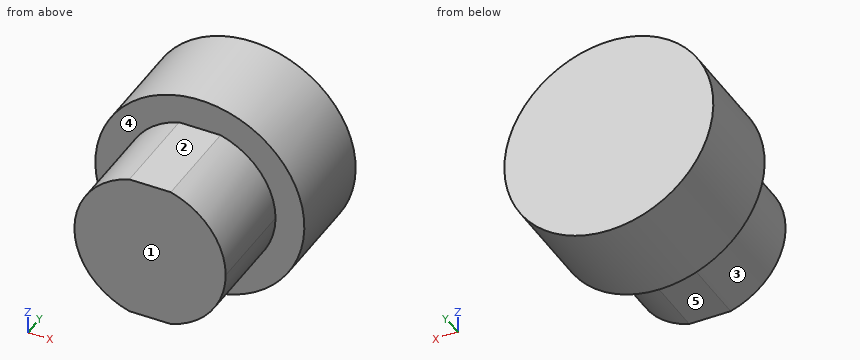
from build123d import *

# Parameters (mm, degrees)
BOSS_EXTRUDE1_DEPTH = 13.3
SKETCH2_R           = 14.5
BOSS_EXTRUDE2_DEPTH = 13.7


with BuildPart() as part:
    # Sketch1 → Boss-Extrude1 (new body)
    with BuildSketch(Plane(origin=(0, 0, 0), x_dir=(1, 0, 0), z_dir=(0, 1, 0))):
        with BuildLine():
            Line((2.870540019, 10.1), (-2.870540019, 10.1))
            ThreePointArc((-2.870540019, 10.1), (-10.5, 0), (-2.870540019, -10.1))
            Line((-2.870540019, -10.1), (2.870540019, -10.1))
            Line((2.870540019, -10.1), (2.870540019, 10.1))
        make_face()
        with BuildLine():
            ThreePointArc((10.5, 0), (8.378265638, 6.328875485), (2.870540019, 10.1))
            Line((2.870540019, 10.1), (2.870540019, -10.1))
            ThreePointArc((2.870540019, -10.1), (8.378265638, -6.328875485), (10.5, 0))
        make_face()
    extrude(amount=BOSS_EXTRUDE1_DEPTH)

    # Sketch2 → Boss-Extrude2 (add)
    with BuildSketch(Plane(origin=(0, 13.3, 0), x_dir=(1, 0, 0), z_dir=(0, 1, 0))):
        with Locations(Location((0, 0, 0), (0, 0, 90))):
            Circle(SKETCH2_R)
    extrude(amount=BOSS_EXTRUDE2_DEPTH)


solid = part.part
Can you work these out from the model? Positions are in its coordinate system, mm. Face numbers are marked on the shaded views. A direction names the side the tool comes from. Round coordinates to 2 decimals unless told otherwise and drop trailing zeros. Order: outer loops, then holes, each group sorted by start corner. A loop starts at its lowest first (then second) coordinate and runs counter-clockwise, first axis right, second up. Notation, with made-up numbers: M 42,34 L 65,34 A11 cw 65,53 Z; hole C 11.25,15 d9. An arc over 180 degrees is marked long. Use a Markdown table: item, result.
1) Imagine slicing it at D-D (y = 19). List the corners of the cut face in (x, z) for me, then the cut area to 3 significant figures.
Geometry says:
| item | result |
|---|---|
| outline | C 0,0 d29 |
| area | 661 mm² |
2) Imagine slicing it at C-C (y = 3.75). List the corners of the cut face in (x, z) for me, then the cut area to 3 significant figures.
Geometry says:
| item | result |
|---|---|
| outline | M -2.87,-10.1 L 2.87,-10.1 A10.5 ccw 2.87,10.1 L -2.87,10.1 A10.5 ccw Z |
| area | 343 mm² |
3) I'm going to push flat-ended pins straight in: P1, Ø10, axis at y = 7, z = 8, coming from the +X side; P2, Ø6.5, axis at x = 1, y = 4, coming from the -Z side; P3, Ø2, axis at y = 4, z = -4.5, coming from the +X side. Where does each tip first touch, or does it pass through?
Geometry says:
| item | result |
|---|---|
| P1 | stops at x = 10.06 |
| P2 | stops at z = -10.1 |
| P3 | stops at x = 9.9 |
4) If I drill on line 1 along Y through (x, z) = (7.25, 10.75); line 2 along Z through (x, y) = (1.75, 5.5); line 3 along X through (y, z) = (10.75, 0), over which ranges is the centre line in solid material (lowest first)?
Geometry says:
| item | result |
|---|---|
| line 1 | y = 13.3 to 27 |
| line 2 | z = -10.1 to 10.1 |
| line 3 | x = -10.5 to 10.5 |
5) Imagine slicing it at B-B (z = -6.5). List the corners of the cut face in (x, y) for me, then the cut area to 3 significant figures.
Geometry says:
| item | result |
|---|---|
| outline | M -12.96,13.3 L -8.25,13.3 L -8.25,0 L 8.25,0 L 8.25,13.3 L 12.96,13.3 L 12.96,27 L -12.96,27 Z |
| area | 574 mm² |
6) Imagine slicing it at A-A (x = 0). List the corners of the cut face in (y, z) for me, then the cut area to 3 significant figures.
Geometry says:
| item | result |
|---|---|
| outline | M 0,-10.1 L 13.3,-10.1 L 13.3,-14.5 L 27,-14.5 L 27,14.5 L 13.3,14.5 L 13.3,10.1 L 0,10.1 Z |
| area | 666 mm² |
7) On a 3-axis mill with a long thin cutter (end or side, diameter ignored), from which of +Z, -Z, +X, -X, +Y, -Y can I reach the whole of each face in a straight line? I mean the marked faces 1, 2, 3, 4 and 5. Say none if no direction works.
Geometry says:
| item | result |
|---|---|
| face 1 | +Z, -Z, +X, -X, -Y |
| face 2 | +Z, +X, -X, -Y |
| face 3 | -X, -Y |
| face 4 | -Y |
| face 5 | -Z, +X, -X, -Y |
